from build123d import *

# Parameters (mm, degrees)
F0_W     = 15
F0_H     = 1
F0_H_2   = 1.2
F0_W_2   = 1.1
F0_H_3   = 6
F0_W_3   = 0.9
F5_DEPTH = 6
F6_R     = 1
F7_R     = 0.3


with BuildPart() as f2:
    # F2: sweep along a path in F1
    with BuildLine(Plane.XZ) as f2_path:
        Line((0, 0), (0, 0.4))
    # F0 (on Top) → F2 (sweep)
    with BuildSketch(Plane.XY):
        Polygon((-10.75, 1), (-10.75, 0), (-7.5, 0), (7.5, 0), (10.75, 0), (10.75, 1), align=None)
        Polygon((-12, 0), (-10.75, 0), (-10.75, 1), (-10.75, 2), (-12, 2), align=None)
        with Locations((0, -0.5)):
            Rectangle(F0_W, F0_H)
        Polygon((-10.75, 2), (-10.75, 1), (10.75, 1), (10.75, 2), (10.75, 10.5), (10.75, 16.5), (-10.75, 16.5), (-10.75, 10.5), align=None)
        with Locations((0, -1.6)):
            Rectangle(F0_W, F0_H_2)
        Polygon((10.75, 2), (10.75, 1), (10.75, 0), (12, 0), (12, 2), align=None)
        with Locations((-11.3, 13.5)):
            Rectangle(F0_W_2, F0_H_3)
        with Locations((-12.3, 13.5)):
            Rectangle(F0_W_3, F0_H_3)
        with Locations((11.3, 13.5)):
            Rectangle(F0_W_2, F0_H_3)
        with Locations((12.3, 13.5)):
            Rectangle(F0_W_3, F0_H_3)
    sweep(path=f2_path.line)

    # F3: sweep along a path in F1
    with BuildLine(Plane.XZ) as f3_path:
        Line((0, 0), (0, 0.4))
        Line((0, 0.4), (0, 2.4))
    # F0 (on Top) → F3 (sweep)
    with BuildSketch(Plane.XY):
        with Locations((12.3, 13.5)):
            Rectangle(F0_W_3, F0_H_3)
        with Locations((-12.3, 13.5)):
            Rectangle(F0_W_3, F0_H_3)
    sweep(path=f3_path.line)

    # F4 (on face) → F5 (join, through all)
    with BuildSketch(Plane(origin=(0, 16.5, 0), x_dir=(-1, 0, 0), z_dir=(0, 1, 0))):
        Polygon((-11.5, 0.4), (-11.85, 2.4), (-11.85, 0.4), align=None)
        Polygon((11.85, 2.4), (11.5, 0.4), (11.85, 0.4), align=None)
    extrude(amount=-F5_DEPTH)

    # F6
    f6_edges = [f2.edges().sort_by_distance(p)[0] for p in [
        (7.5, 0, 0.2),
        (-7.5, 0, 0.2),
        (-10.75, 2, 0.2),
        (-10.75, 10.5, 0.2),
        (10.75, 10.5, 0.2),
        (10.75, 2, 0.2),
    ]]
    fillet(f6_edges, radius=F6_R)

    # F7
    f7_edges = [f2.edges().sort_by_distance(p)[0] for p in [
        (-12.75, 16.5, 1.2),
        (12.75, 16.5, 1.2),
        (12.75, 10.5, 1.2),
        (-12.75, 10.5, 1.2),
    ]]
    fillet(f7_edges, radius=F7_R)


solid = f2.part
Could you check a few things on this model? Use its own coordinates, in mm. A direction names the side the tool comes from. Coordinates: 2 decimals unless noted, no trailing zeros. Order: outer loops, then holes, each group sorted by start corner. A loop starts at its lowest first (then second) coordinate and runs counter-clockwise, first axis right, second up.
Q1. Thinking about a two-plate mould opening in X: for faces 4 (the flat face through (11.673, 13.526, 1.386)), 5 (the flat face through (12.3, 13.5, 2.4)), 6 (the cylindrical face through (-7.785, -0.301, 0.203)), which applies, released by +X, released by -X, zero draft, split by the parting line, or undercut?
Q2. Suppose I cut it at C-C on x = -2. Please give me the cut outline in (y, z), and give its area (3 significant figures).
Q3. Please list where these lines run through material, in increasing order: L1, parallel to Z at x = 3, y = 4; L2, parallel to X at y = 9, z = 0.1; L3, parallel to X at y = 14.5, z = 1.25.
Q4. Which directions (+Z, -Z, +X, -X, +Y, -Y) give clear straight access to the entire face, cutting with the end or side of a thin tool? Please do faces 1 (the flat face through (-11.677, 13.526, 1.414)), 2 (the cylindrical face through (11.18, 10.32, 0.24)), 3 (the cylindrical face through (-11.051, 2.285, 0.203)).
Q5. Suppose I cut it at D-D on y = 3.5. Please give me the cut outline in (x, z), and give its area (3 significant figures).
Q6. Suppose I cut it at A-A on z = 1.5. Please give me the cut outline in (x, y).
Q7. Will these pins go through, and if not, where does the flat tip stop? pin 1 (0.6 mm diameter, centred on x = 12, z = 1, fed in from -Y); pin 2 (5.5 mm diameter, centred on x = -3.5, y = 7.5, fed in from +Z); pin 3 (10 mm diameter, centred on x = 5, y = 6.5, fed in from -Z).
Q8. Suppose I cut it at B-B on y = 11.5. Please give me the cut outline in (x, z), and give its area (3 significant figures).
Answer:
1. face 4: undercut
1. face 5: zero draft
1. face 6: released by -X
2. outline: (-2.2, 0) - (16.5, 0) - (16.5, 0.4) - (-2.2, 0.4) - close
2. area: 7.48 mm2
3. L1: z = 0 to 0.4
3. L2: x = -10.75 to 10.75
3. L3: x = -12.75 to -11.65, 11.65 to 12.75
4. face 1: +Z, +Y, -Y
4. face 2: +Z, -Z, +X
4. face 3: +Z, -Z, -X
5. outline: (-10.75, 0) - (10.75, 0) - (10.75, 0.4) - (-10.75, 0.4) - close
5. area: 8.60 mm2
6. outline: (-12.75, 10.8) arc R0.3 ccw to (-12.45, 10.5) - (-11.75, 10.5) arc R1 cw to (-11.69, 10.5) - (-11.69, 16.5) - (-12.45, 16.5) arc R0.3 ccw to (-12.75, 16.2) - close; (11.69, 10.5) arc R1 cw to (11.75, 10.5) - (12.45, 10.5) arc R0.3 ccw to (12.75, 10.8) - (12.75, 16.2) arc R0.3 ccw to (12.45, 16.5) - (11.69, 16.5) - close
7. pin 1: stops at y = 10.5
7. pin 2: stops at z = 0.4
7. pin 3: stops at z = 0
8. outline: (-12.75, 0) - (12.75, 0) - (12.75, 2.4) - (11.85, 2.4) - (11.5, 0.4) - (-11.5, 0.4) - (-11.85, 2.4) - (-12.75, 2.4) - close
8. area: 14.5 mm2
